from build123d import *

# Parameters (mm, degrees)
F0_R     = 2
F1_DEPTH = 70
F2_R     = 10
F3_DEPTH = 5
F4_R     = 1
F5_R     = 10
F5_R_2   = 2
F6_DEPTH = 5
F7_R     = 1


# Not quite as in the source:
# - a feature names something its author has since deleted; it is built from what else it names


with BuildPart() as f1:
    # F0 (on Front) → F1 (new body)
    with BuildSketch(Plane.XZ):
        Circle(F0_R)
    extrude(amount=F1_DEPTH)

    # F2 (on face) → F3 (join)
    with BuildSketch(Plane.XZ.offset(70)):
        Circle(F2_R)
    extrude(amount=F3_DEPTH)

    # F4
    f4_edges = [f1.edges().sort_by_distance(p)[0] for p in [
        (-10, -70, 0),
        (-10, -75, 0),
    ]]
    fillet(f4_edges, radius=F4_R)

    # F5 (on face) → F6 (join)
    with BuildSketch(Plane(origin=(0, 0, 0), x_dir=(-1, 0, 0), z_dir=(0, 1, 0))):
        Circle(F5_R)
        Circle(F5_R_2, mode=Mode.SUBTRACT)
        Circle(F5_R_2)
    extrude(amount=F6_DEPTH)

    # F7
    f7_edges = [f1.edges().sort_by_distance(p)[0] for p in [
        (10, 0, 0),
        (10, 5, 0),
    ]]
    fillet(f7_edges, radius=F7_R)


solid = f1.part
Design review of the part built by this model. Coordinates are the model's own, in mm. A direction names the side the tool comes from. Give positions to 0.01 mm unless a question says otherwise; leave off trailing zeros. Loops run counter-clockwise (first coordinate to the right, second up) from the corner with the lowest first, then second, coordinate; pieces in that order, holes last. Notation, with made-up numbers: (53.25, 86) -> (59.25, 86) arc R15 ccw to (59.25, 91) -> close; hole circle Ø4 at (-37.75, 77). An arc over 180 degrees is marked (long way). One line per question, with ' | ' between items. Start each with the question number.
(1) For faces 4 (the face through (0, -75, 0)), 5 (the face through (0, -35, -2)), list the 3-axis set-ups (+Z, -Z, +X, -X, +Y, -Y) from which the entire face can be reached by the end or side of a thin tool; tool diameter is ignored.
(2) Insertion check: P1, Ø1.5, axis at y = -35, z = -3, coming from the +X side; P2, Ø12, axis at x = 3, y = -12, coming from the +Z side; P3, Ø12, axis at x = 0, y = -19.5, coming from the -Z side; P4, Ø2, axis at y = -55.5, z = -2.5, coming from the -X side. Each pin has a flat end and moves straight along its axis. Give the tip position at first contact, or say it passes through.
(3) We need section C-C (y = -10.5). State the section outline as (x, z) points.
(4) We need section B-B (x = 0). State the section outline as (y, z) points, and give its area (3 significant figures).
(5) For line 1 (Y direction, x = -6.5, z = -3); line 2 (Z direction, x = 0, y = -44); line 3 (X direction, y = -35.5, z = 0.25), list the stretches that pass through material, from the lowest coordinate up.
(6) We need section A-A (z = 0). State the section outline as (x, y) points.
(7) Draft analysis for pull direction Y (two halves, no side actions). For faces 1 (the face through (0, 5, 0)), 2 (the face through (-2, 0, -2)), 3 (the face through (-2.17, -72.48, -9.76)), state which applies: +Y half, -Y half, draft (parallel to the pull), parting line (faces both ways), or undercut.
The answers:
1) face 4: +Z, -Z, +X, -X, -Y | face 5: none
2) P1: passes through | P2: stops at z = 2 | P3: stops at z = -2 | P4: stops at x = -1.32
3) outline: circle Ø4 at (0, 0)
4) outline: (-75, -9) arc R1 ccw to (-74, -10) -> (-71, -10) arc R1 ccw to (-70, -9) -> (-70, -2) -> (0, -2) -> (0, -9) arc R1 ccw to (1, -10) -> (4, -10) arc R1 ccw to (5, -9) -> (5, 9) arc R1 ccw to (4, 10) -> (1, 10) arc R1 ccw to (0, 9) -> (0, 2) -> (-70, 2) -> (-70, 9) arc R1 ccw to (-71, 10) -> (-74, 10) arc R1 ccw to (-75, 9) -> close | area: 478 mm^2
5) line 1: y = -75 to -70, 0 to 5 | line 2: z = -2 to 2 | line 3: x = -1.98 to 1.98
6) outline: (-10, -74) arc R1 ccw to (-9, -75) -> (9, -75) arc R1 ccw to (10, -74) -> (10, -71) arc R1 ccw to (9, -70) -> (2, -70) -> (2, 0) -> (9, 0) arc R1 ccw to (10, 1) -> (10, 4) arc R1 ccw to (9, 5) -> (-9, 5) arc R1 ccw to (-10, 4) -> (-10, 1) arc R1 ccw to (-9, 0) -> (-2, 0) -> (-2, -70) -> (-9, -70) arc R1 ccw to (-10, -71) -> close
7) face 1: +Y half | face 2: undercut | face 3: draft
